The model under review builds one solid part; all positions refer to its coordinate system, in mm. Round coordinates to 2 decimals unless told otherwise and drop trailing zeros. Loops run counter-clockwise (first coordinate to the right, second up) from the corner with the lowest first, then second, coordinate; pieces in that order, holes last. Notation, with made-up numbers: M 45.25,38.5 L 74.25,38.5 A28 ccw 74.25,76.5 Z; hole C 73.5,49.25 d11. An arc over 180 degrees is marked long. Answer as a JSON object with one key per item and string values. Group by question number.
Item 1: Consider section C-C (x = -8). Give the boundary of the cut face in (y, z) (3 decimals).
Item 2: Insertion check: P1, Ø3.5, axis at x = -38.1, z = 0, coming from the +Y side; P2, Ø1, axis at x = -2.5, y = 0, coming from the +Z side; P3, Ø0.5, axis at y = 0.5, z = 41, coming from the -X side; P4, Ø0.5, axis at y = 0.5, z = 25, coming from the -X side. Each pin has a flat end and moves straight along its axis. Give the tip position at first contact, or say it passes through.
Item 3: Consider section B-B (z = 25.4). Give the boundary of the cut face in (x, y) (3 decimals).
Item 4: Consider section D-D (z = 32.5). Give the boundary of the cut face in (x, y) (3 decimals), and give its area (3 significant figures).
Item 5: Consider section A-A (x = -63.5). Give the boundary of the cut face in (y, z) (3 decimals).
Item 6: To check wall thickness, follow line 1 (Z direction, x = -18, y = -0.1); line 2 (Z direction, x = -38, y = 0.7); line 3 (X direction, y = -0.6, z = 37). State the ranges of each line that lie inside material, in increasing order.
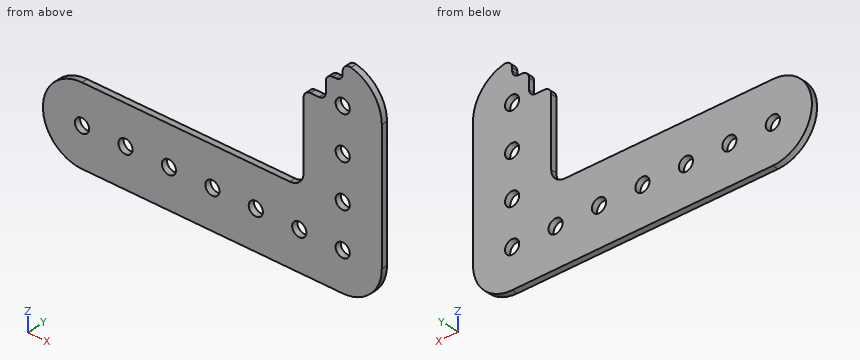
```python
from build123d import *

# Parameters (mm, degrees)
SKETCH1_R               = 2.07
BOSS_EXTRUDE1_DEPTH     = 0.875
FILLET1_R               = 4
CUT_EXTRUDE3_DEPTH      = 101.674228579
CUT_EXTRUDE3_DEPTH_BACK = 101.674228579
CUT_EXTRUDE4_DEPTH      = 101.674228579
CUT_EXTRUDE4_DEPTH_BACK = 101.674228579
FILLET3_R               = 2


with BuildPart() as part:
    # Sketch1 → Boss-Extrude1 (new, symmetric)
    with BuildSketch(Plane(origin=(0, 0, 0), x_dir=(1, 0, 0), z_dir=(0, 1, 0))):
        with BuildLine():
            Line((0, 11.43), (-76.2, 11.43))
            ThreePointArc((-76.2, 11.43), (-87.63, 0), (-76.2, -11.43))
            Line((-76.2, -11.43), (-11.43, -11.43))
            Line((-11.43, -11.43), (-11.43, -38.1))
            ThreePointArc((-11.43, -38.1), (0, -49.53), (11.43, -38.1))
            Line((11.43, -38.1), (11.43, 0))
            ThreePointArc((11.43, 0), (8.082230509, 8.082230509), (0, 11.43))
        make_face()
        with Locations(Location((0, -25.4, 0), (0, 0, 270))):
            Circle(SKETCH1_R, mode=Mode.SUBTRACT)
        with Locations(Location((0, -12.7, 0), (0, 0, 270))):
            Circle(SKETCH1_R, mode=Mode.SUBTRACT)
        with Locations(Location((-12.7, 0, 0), (0, 0, 270))):
            Circle(SKETCH1_R, mode=Mode.SUBTRACT)
        with Locations(Location((-63.5, 0, 0), (0, 0, 270))):
            Circle(SKETCH1_R, mode=Mode.SUBTRACT)
        with Locations(Location((-50.8, 0, 0), (0, 0, 270))):
            Circle(SKETCH1_R, mode=Mode.SUBTRACT)
        with Locations(Location((-38.1, 0, 0), (0, 0, 270))):
            Circle(SKETCH1_R, mode=Mode.SUBTRACT)
        with Locations(Location((-25.4, 0, 0), (0, 0, 270))):
            Circle(SKETCH1_R, mode=Mode.SUBTRACT)
        with Locations(Location((-76.2, 0, 0), (0, 0, 270))):
            Circle(SKETCH1_R, mode=Mode.SUBTRACT)
        with Locations(Location((0, 0, 0), (0, 0, 270))):
            Circle(SKETCH1_R, mode=Mode.SUBTRACT)
        with Locations(Location((0, -38.1, 0), (0, 0, 270))):
            Circle(SKETCH1_R, mode=Mode.SUBTRACT)
    extrude(amount=BOSS_EXTRUDE1_DEPTH, both=True)

    # Fillet1
    fillet1_edges = [part.edges().sort_by_distance(p)[0] for p in [
        (-11.43, 0, 11.43),
    ]]
    fillet(fillet1_edges, radius=FILLET1_R)

    # Sketch4 → Cut-Extrude3 (cut, two sides: drawn at the far end of the back side and taken through both)
    with BuildSketch(Plane(origin=(0, 0.875, 0), x_dir=(1, 0, 0), z_dir=(0, 1, 0)).offset(-CUT_EXTRUDE3_DEPTH_BACK)):
        with BuildLine():
            Line((-4.93, -37.43), (-4.93, -48.412128781))
            ThreePointArc((-4.93, -48.412128781), (-9.669405359, -44.194874896), (-11.43, -38.1))
            Line((-11.43, -38.1), (-11.43, -37.43))
            Line((-11.43, -37.43), (-4.93, -37.43))
        make_face()
    extrude(amount=CUT_EXTRUDE3_DEPTH + CUT_EXTRUDE3_DEPTH_BACK, mode=Mode.SUBTRACT)

    # Sketch5 → Cut-Extrude4 (cut, two sides: drawn at the far end of the back side and taken through both)
    with BuildSketch(Plane(origin=(0, 0.875, 0), x_dir=(1, 0, 0), z_dir=(0, 1, 0)).offset(-CUT_EXTRUDE4_DEPTH_BACK)):
        with BuildLine():
            Line((-4.93, -44.53), (0, -44.53))
            Line((0, -44.53), (0, -49.53))
            ThreePointArc((0, -49.53), (-2.52757473, -49.247029469), (-4.93, -48.412128781))
            Line((-4.93, -48.412128781), (-4.93, -44.53))
        make_face()
    extrude(amount=CUT_EXTRUDE4_DEPTH + CUT_EXTRUDE4_DEPTH_BACK, mode=Mode.SUBTRACT)

    # Fillet3
    fillet3_edges = [part.edges().sort_by_distance(p)[0] for p in [
        (0, 0, 49.53),
        (0, 0, 44.53),
        (-4.93, 0, 44.53),
        (-4.93, 0, 37.43),
        (-11.43, 0, 37.43),
    ]]
    fillet(fillet3_edges, radius=FILLET3_R)


solid = part.part
```
Geometry results:
{
 "1": {"outline": "M -0.875,-11.43 L 0.875,-11.43 L 0.875,37.43 L -0.875,37.43 Z"},
 "2": {"P1": "passes through", "P2": "stops at z = 44.53", "P3": "stops at x = -4.93", "P4": "stops at x = -11.43"},
 "3": {"outline": "M -11.43,-0.875 L -2.07,-0.875 L -2.07,0.875 L -11.43,0.875 Z; M 2.07,-0.875 L 11.43,-0.875 L 11.43,0.875 L 2.07,0.875 Z"},
 "4": {"outline": "M -11.43,-0.875 L 11.43,-0.875 L 11.43,0.875 L -11.43,0.875 Z", "area": "40.0 mm^2"},
 "5": {"outline": "M -0.875,-11.43 L 0.875,-11.43 L 0.875,-2.07 L -0.875,-2.07 Z; M -0.875,2.07 L 0.875,2.07 L 0.875,11.43 L -0.875,11.43 Z"},
 "6": {"line 1": "z = -11.43 to 11.43", "line 2": "z = -11.43 to -2.07, 2.07 to 11.43", "line 3": "x = -10.67 to -1.75, 1.75 to 11.43"}
}
